Solid Edge part; units mm, degrees
sketch "Sketch1" plane through (0, 0, 0) normal (0, -1, 0) x (1, 0, 0)
  line L0 (22.5, 36.5) -> (22.5, -33)
  line L1 (22.5, -33) -> (-22.5, -33)
  line L2 (-22.5, -33) -> (-22.5, 36.5)
  line L3 (-22.5, 36.5) -> (22.5, 36.5)
  circle A0 centre (0, 28) radius 6
  circle A1 centre (0, 8) radius 4.6
  circle A2 centre (-17.5, 0) radius 2
  circle A3 centre (17.5, 0) radius 2
extrude "Protrusion1" add sketch "Sketch1" against normal blind 10
sketch "Sketch2" plane through (0, 10, 4.6) normal (0, 1, 0) x (-1, 0, 0)
  circle A0 centre (0, 3.4) radius 11.25
extrude "ExtrudedCutout_1" cut sketch "Sketch2" against normal blind 7.5
sketch "Sketch3" plane through (0, 5, -33) normal (0, 0, -1) x (1, 0, 0)
  circle A0 centre (-17.5, 0) radius 2.5
  circle A1 centre (17.5, 0) radius 2.5
extrude "ExtrudedCutout_2" cut sketch "Sketch3" against normal blind 10
sketch "Sketch4" plane through (0, 0, 0) normal (0, -1, 0) x (1, 0, 0)
  line L0 (-22.5, 36.5) -> (22.5, 36.5)
  line L1 (22.5, 36.5) -> (22.5, -33)
  line L2 (22.5, -33) -> (-22.5, -33)
  line L3 (-22.5, -33) -> (-22.5, 36.5)
  circle A0 centre (0, 8) radius 4.6
  circle A1 centre (0, 28) radius 6
  circle A2 centre (-17.5, 0) radius 2
  circle A3 centre (17.5, 0) radius 2
extrude "ExtrudedProtrusion_2" add sketch "Sketch4" along normal blind 1.7
sketch "Sketch5" plane through (0, 10, 3.5) normal (0, 1, 0) x (-1, 0, 0)
  circle A0 centre (-17.5, 22) radius 1.5
  circle A1 centre (-17.5, 2) radius 1.5
extrude "Cutout1" cut sketch "Sketch5" against normal up to next
Verification items for the finished model (mm, model axes). A direction names the side the tool comes from. Coordinates: 2 decimals unless noted, no trailing zeros. Loops run counter-clockwise (first coordinate to the right, second up) from the corner with the lowest first, then second, coordinate; pieces in that order, holes last. Notation, with made-up numbers: (30, 4) - (77, 4) arc R16 cw to (77, 17) - close; hole circle Ø1 at (43, 31.25). An arc over 180 degrees is marked (long way). Put each result on its own line as item: value.
Item 1: Draft check along Y on faces 4 (the face through (18, 5, -23)), 5 (the face through (0, -1.7, 1)), 6 (the face through (22.5, 4, 2)), 7 (the face through (-5, 2.5, 8)). Enter one of: pulls with the +Y half, pulls with the -Y half, needs draft (parallel to the pull), parting line crosses it, or undercut.
Conclusion:
face 4: undercut
face 5: pulls with the -Y half
face 6: needs draft
face 7: pulls with the +Y half
Item 2: Section check B-B (z = 28). Enter the section's corners in (x, y), then the cut area to 3 significant figures.
Conclusion:
outline: (-22.5, -1.7) - (-6, -1.7) - (-6, 10) - (-22.5, 10) - close; (6, -1.7) - (22.5, -1.7) - (22.5, 10) - (6, 10) - close
area: 386 mm2
Item 3: Scan lines: line 1 along X through (y, z) = (5, -27.5); line 2 along Z through (x, y) = (0, -0.4); line 3 along Z through (x, y) = (-3, 8.25). Record each from-to range of solid material in increasing order.
Conclusion:
line 1: x = -22.5 to -20, -15 to 15, 20 to 22.5
line 2: z = -33 to 3.4, 12.6 to 22, 34 to 36.5
line 3: z = -33 to -2.84, 18.84 to 22.8, 33.2 to 36.5
Item 4: Set-up check for faces 1 (the face through (19, 4.23, 5.57)), 2 (the face through (2.439, 6.302, -2.982)), 3 (the face through (-17, 5, -23)): record each of +Z, -Z, +X, -X, +Y, -Y from which the full face is reachable in a straight line by a thin tool's end or side.
Conclusion:
face 1: +Y, -Y
face 2: +Y
face 3: -Z
Item 5: Section check A-A (x = -17.5). Enter the section's corners in (y, z).
Conclusion:
outline: (-1.7, -33) - (2.5, -33) - (2.5, -23) - (7.5, -23) - (7.5, -33) - (10, -33) - (10, -2) - (-1.7, -2) - close; (-1.7, 2) - (10, 2) - (10, 36.5) - (-1.7, 36.5) - close
Item 6: Section check D-D (y = 3.75). Enter the section's corners in (x, z), then the cut area to 3 significant figures.
Conclusion:
outline: (-22.5, -33) - (-19.67, -33) - (-19.67, -23) - (-15.33, -23) - (-15.33, -33) - (15.33, -33) - (15.33, -23) - (19.67, -23) - (19.67, -33) - (22.5, -33) - (22.5, 36.5) - (-22.5, 36.5) - close; hole circle Ø4 at (-17.5, 0); hole circle Ø22.5 at (0, 8); hole circle Ø12 at (0, 28); hole circle Ø4 at (17.5, 0); hole circle Ø3 at (17.5, 5.5); hole circle Ø3 at (17.5, 25.5)
area: 2,490 mm2
Item 7: Section check C-C (x = 0). Enter the section's corners in (y, z), then the cut area to 3 significant figures.
Conclusion:
outline: (-1.7, -33) - (10, -33) - (10, -3.25) - (2.5, -3.25) - (2.5, 3.4) - (-1.7, 3.4) - close; (-1.7, 12.6) - (2.5, 12.6) - (2.5, 19.25) - (10, 19.25) - (10, 22) - (-1.7, 22) - close; (-1.7, 34) - (10, 34) - (10, 36.5) - (-1.7, 36.5) - close
area: 465 mm2
